Read the model definition and answer for the solid it produces. Units are mm, in the model's axes. A direction names the side the tool comes from. Give positions to 0.01 mm unless a question says otherwise; leave off trailing zeros. Order: outer loops, then holes, each group sorted by start corner. A loop starts at its lowest first (then second) coordinate and runs counter-clockwise, first axis right, second up. Notation, with made-up numbers: (35.5, 13.25) - (41.5, 13.25) arc R23 cw to (41.5, 38.25) - close; hole circle Ø2 at (87.5, -27). An arc over 180 degrees is marked (long way). Write each question's results on one line, items separated by ' | '.
from build123d import *

# Parameters (mm, degrees)
BOSS_EXTRUDE1_DEPTH = 6.35
SKETCH2_R           = 6.35
CUT_EXTRUDE1_DEPTH  = 6.35
CUT_EXTRUDE3_DEPTH  = 6.35
CUT_EXTRUDE4_DEPTH  = 6.35
CUT_EXTRUDE6_DEPTH  = 6.35


with BuildPart() as part:
    # Sketch1 → Boss-Extrude1 (new body)
    with BuildSketch(Plane.XY):
        Polygon((20.505148302, 25.897062134), (-23.613528139, 31.314154449), (25.914173021, 434.684910476), (95.764173021, 434.684910476), (95.764173021, 95.747062134), (29.081649881, 95.747062134), align=None)
    extrude(amount=BOSS_EXTRUDE1_DEPTH)

    # Sketch2 → Cut-Extrude1 (cut)
    with BuildSketch(Plane.XY.offset(6.35)):
        with Locations((72.594859494, 436.135448726)):
            Circle(SKETCH2_R)
    extrude(amount=-CUT_EXTRUDE1_DEPTH, mode=Mode.SUBTRACT)

    # Sketch3 → Cut-Extrude3 (cut)
    with BuildSketch(Plane.XY.offset(6.35)):
        with BuildLine():
            ThreePointArc((59.06996097, 226.736339707), (66.497801827, 244.661042374), (63.213102929, 263.783765471))
            ThreePointArc((63.213102929, 263.783765471), (54.728545327, 266.726091472), (51.786219326, 258.24153387))
            ThreePointArc((51.786219326, 258.24153387), (53.876482261, 246.072528262), (49.149674443, 234.665899293))
            ThreePointArc((49.149674443, 234.665899293), (50.145037914, 225.740976236), (59.06996097, 226.736339707))
        make_face()
    extrude(amount=-CUT_EXTRUDE3_DEPTH, mode=Mode.SUBTRACT)

    # Sketch4 → Cut-Extrude4 (cut)
    with BuildSketch(Plane.XY.offset(6.35)):
        with BuildLine():
            Line((74.295018445, 431.943320697), (82.016159891, 440.361424689))
            Line((82.016159891, 440.361424689), (105.989857785, 438.164600241))
            Line((105.989857785, 438.164600241), (95.764173021, 334.935994434))
            ThreePointArc((95.764173021, 334.935994434), (92.231289046, 356.088107858), (82.016159891, 374.943990437))
            ThreePointArc((82.016159891, 374.943990437), (70.461962448, 402.401475249), (74.295018445, 431.943320697))
        make_face()
    extrude(amount=-CUT_EXTRUDE4_DEPTH, mode=Mode.SUBTRACT)

    # Sketch5 → Cut-Extrude6 (cut)
    with BuildSketch(Plane.XY.offset(6.35)):
        with BuildLine():
            Line((26.231673021, 287.120128567), (37.026673021, 287.120128567))
            ThreePointArc((37.026673021, 287.120128567), (41.516801082, 285.260256628), (43.376673021, 280.770128567))
            Line((43.376673021, 280.770128567), (43.376673021, 236.955128567))
            ThreePointArc((43.376673021, 236.955128567), (41.516801082, 232.465000507), (37.026673021, 230.605128567))
            Line((37.026673021, 230.605128567), (26.231673021, 230.605128567))
            ThreePointArc((26.231673021, 230.605128567), (21.74154496, 232.465000507), (19.881673021, 236.955128567))
            Line((19.881673021, 236.955128567), (19.881673021, 280.770128567))
            ThreePointArc((19.881673021, 280.770128567), (21.74154496, 285.260256628), (26.231673021, 287.120128567))
        make_face()
    extrude(amount=-CUT_EXTRUDE6_DEPTH, mode=Mode.SUBTRACT)


solid = part.part
(1) Section A-A (y = 251.5) is taken. Give the vertices of the cut face in (x, z).
Conclusion:
outline: (3.42, 0) - (19.88, 0) - (19.88, 6.35) - (3.42, 6.35) - close; (43.38, 0) - (53.82, 0) - (53.82, 6.35) - (43.38, 6.35) - close; (66.59, 0) - (95.76, 0) - (95.76, 6.35) - (66.59, 6.35) - close
(2) Section D-D (y = 124) is taken. Give the vertices of the cut face in (x, z), plus the area to 3 significant figures.
Conclusion:
outline: (-12.23, 0) - (95.76, 0) - (95.76, 6.35) - (-12.23, 6.35) - close | area: 686 mm^2
(3) The mould has two halves that part along Y. Classify faces 3 (the face through (54.855, 266.786, 3.219)), 4 (the face through (50.037, 225.829, 3.219)), 5 (the face through (92.33, 355.8, 3.22)), 6 (the face through (24.853, 61.311, 3.131)): pulls with the +Y half, pulls with the -Y half, needs draft (parallel to the pull), parting line crosses it, or undercut.
Conclusion:
face 3: undercut | face 4: undercut | face 5: pulls with the +Y half | face 6: pulls with the -Y half
(4) Each of these flat-tipped pins is pushed along its axis until it touches: pin 1 (3 mm diameter, centred on x = 73.5, z = 5, fed in from -Y); pin 2 (1 mm diameter, centred on y = 248.5, z = 4.5, fed in from -X); pin 3 (1.9 mm diameter, centred on y = 256, z = 3.5, fed in from -X). Where does it stop, or does it pass through?
Conclusion:
pin 1: y = 95.75 | pin 2: x = 2.99 | pin 3: x = 3.86
(5) Consider probe 1 along X at (y, z) = (387.5, 2.75); probe 2 along X at (y, z) = (100, 1); probe 3 along Y at (x, z) = (61, 3.5). Determine where each line is inside the solid, lowest interval first. Write a range as [from, to].
Conclusion:
probe 1: [20.12, 74.59] | probe 2: [-15.18, 95.76] | probe 3: [95.75, 229.4], [266.31, 434.68]
(6) Section C-C (x = 85.5) is taken. Give the vertices of the cut face in (y, z), plus the area to 3 significant figures.
Conclusion:
outline: (95.75, 0) - (370.02, 0) - (370.02, 6.35) - (95.75, 6.35) - close | area: 1,740 mm^2
(7) Section B-B (z = 5) is taken. State how many separate pieces and enclosed holes the cut face has, plus the area to 3 significant figures.
Conclusion:
separate pieces: 1 | enclosed holes: 2 | area: 30,300 mm^2
(8) For faces 1 (the face through (0.804, 230.176, 3.131)), 2 (the face through (66.466, 244.388, 3.219)), determine the directions among +Z, -Z, +X, -X, +Y, -Y from which every point of the face is accessible in a straight line to the end or side of a thin tool.
Conclusion:
face 1: +Z, -Z, -X, +Y | face 2: +Z, -Z
